For this review, take the finished solid that the model builds, in its own axes (mm). Face numbers are marked on the shaded views. A direction names the side the tool comes from. Coordinates: 2 decimals unless noted, no trailing zeros. Loops run counter-clockwise (first coordinate to the right, second up) from the corner with the lowest first, then second, coordinate; pieces in that order, holes last. Notation, with made-up numbers: (73.5, 33) -> (112.5, 33) arc R19 ccw to (112.5, 37) -> close; hole circle Ø9 at (79, -19.75). An arc over 180 degrees is marked (long way). Use a Markdown table: item, result.
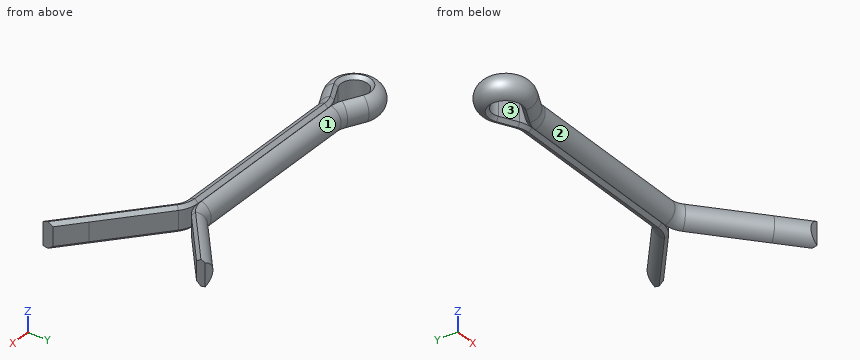
from build123d import *

# Parameters (mm, degrees)
ZKOSIT1_SIZE                  = 0.257142857
ZKOSIT2_SIZE                  = 0.45
ODEBRAT_VYSUNUT_M2_DEPTH      = 10
ODEBRAT_VYSUNUT_M2_DEPTH_BACK = 10
ODEBRAT_VYSUNUT_M3_DEPTH      = 15.066370457
ODEBRAT_VYSUNUT_M3_DEPTH_BACK = 15.066370457


with BuildPart() as part:
    # Táhnout po křivce1: sweep along a path in Skica1
    with BuildLine(Plane.XY) as t_hnout_po_k_ivce1_path:
        Line((10.498702419, 4.371053092), (6.640879802, 1.133955557))
        ThreePointArc((6.640879802, 1.133955557), (6.340112335, 0.960307379), (5.998092192, 0.9))
        Line((5.998092192, 0.9), (-5.998092192, 0.9))
        ThreePointArc((-5.998092192, 0.9), (-6.231322977, 0.927578589), (-6.451689409, 1.008793198))
        Line((-6.451689409, 1.008793198), (-7.621462583, 1.604172244))
        ThreePointArc((-7.621462583, 1.604172244), (-10.237937574, 0), (-7.621462583, -1.604172244))
        Line((-7.621462583, -1.604172244), (-6.451689409, -1.008793198))
        ThreePointArc((-6.451689409, -1.008793198), (-6.231322977, -0.927578589), (-5.998092192, -0.9))
        Line((-5.998092192, -0.9), (5.998092192, -0.9))
        ThreePointArc((5.998092192, -0.9), (6.340112335, -0.960307379), (6.640879802, -1.133955557))
        Line((6.640879802, -1.133955557), (10.498702419, -4.371053092))
        Line((10.498702419, -4.371053092), (12.413813527, -5.978022117))
    # Skica2 → Táhnout po křivce1 (sweep)
    with BuildSketch(Plane(origin=(10.498702419, 4.371053092, 0), x_dir=(0, 0, -1), z_dir=(0.7660444431189762, 0.6427876096865417, 0))):
        with BuildLine():
            Line((0.9, -0.9), (-0.9, -0.9))
            ThreePointArc((-0.9, -0.9), (0, 0), (0.9, -0.9))
        make_face()
    sweep(path=t_hnout_po_k_ivce1_path.line)

    # Zkosit1
    # the kernel refuses this chamfer: 0.257142857 mm, written as the material it takes off along each edge
    with BuildSketch(Plane(origin=(5.998092192, 0, 0.9), x_dir=(0, 0, -1), z_dir=(-1, 0, 0)), Plane(origin=(-5.998092192, 0, 0.9), x_dir=(0, 0, -1), z_dir=(1, 0, 0))) as zkosit1_piece_1:
        with BuildLine():
            Line((ZKOSIT1_SIZE, 0), (0.029314045, -0.227828812))
            ThreePointArc((0.029314045, -0.227828812), (0.007766605, -0.117981219), (0, 0))
            Line((0, 0), (ZKOSIT1_SIZE, 0))
        make_face()
    extrude(amount=11.996184384, mode=Mode.SUBTRACT)
    with BuildSketch(Plane(origin=(5.998092192, 0, -0.9), x_dir=(0, 0, 1), z_dir=(-1, 0, 0)), Plane(origin=(-5.998092192, 0, -0.9), x_dir=(0, 0, 1), z_dir=(1, 0, 0))) as zkosit1_piece_2:
        with BuildLine():
            Line((ZKOSIT1_SIZE, 0), (0.029314045, 0.227828812))
            ThreePointArc((0.029314045, 0.227828812), (0.007766605, 0.117981219), (0, 0))
            Line((0, 0), (ZKOSIT1_SIZE, 0))
        make_face()
    extrude(amount=11.996184384, mode=Mode.SUBTRACT)
    with BuildSketch(Plane(origin=(-5.998092192, 1.9, 0.9), x_dir=(0, -1, 0), z_dir=(1, 0, 0))) as zkosit1_piece_3:
        with BuildLine():
            Line((1.9, ZKOSIT1_SIZE), (1.672171188, 0.029314045))
            ThreePointArc((1.672171188, 0.029314045), (1.782018781, 0.007766605), (1.9, 0))
            Line((1.9, 0), (1.9, ZKOSIT1_SIZE))
        make_face()
    revolve(axis=Axis((-5.998092192, 1.9, 0.9), (0, 0, -1)), revolution_arc=26.974712985, mode=Mode.SUBTRACT)
    with BuildSketch(Plane(origin=(-5.998092192, 1.9, -0.9), x_dir=(0, -1, 0), z_dir=(1, 0, 0))) as zkosit1_piece_4:
        with BuildLine():
            Line((1.9, -ZKOSIT1_SIZE), (1.672171188, -0.029314045))
            ThreePointArc((1.672171188, -0.029314045), (1.782018781, -0.007766605), (1.9, 0))
            Line((1.9, 0), (1.9, -ZKOSIT1_SIZE))
        make_face()
    revolve(axis=Axis((-5.998092192, 1.9, -0.9), (0, 0, -1)), revolution_arc=26.974712985, mode=Mode.SUBTRACT)
    with BuildSketch(Plane(origin=(-6.859926905, 0.206707076, 0.9), x_dir=(0, 0, -1), z_dir=(-0.8912068023322748, 0.4535972172276652, 0)), Plane(origin=(-8.029700078, -0.802086122, 0.9), x_dir=(0, 0, -1), z_dir=(0.8912068023322748, 0.45359721722766544, 0))) as zkosit1_piece_5:
        with BuildLine():
            Line((ZKOSIT1_SIZE, 0), (0.029314045, -0.227828812))
            ThreePointArc((0.029314045, -0.227828812), (0.007766605, -0.117981219), (0, 0))
            Line((0, 0), (ZKOSIT1_SIZE, 0))
        make_face()
    extrude(amount=1.312572088, mode=Mode.SUBTRACT)
    with BuildSketch(Plane(origin=(-6.859926905, 0.206707076, -0.9), x_dir=(0, 0, 1), z_dir=(-0.8912068023322748, 0.4535972172276652, 0)), Plane(origin=(-8.029700078, -0.802086122, -0.9), x_dir=(0, 0, 1), z_dir=(0.8912068023322748, 0.45359721722766544, 0))) as zkosit1_piece_6:
        with BuildLine():
            Line((ZKOSIT1_SIZE, 0), (0.029314045, 0.227828812))
            ThreePointArc((0.029314045, 0.227828812), (0.007766605, 0.117981219), (0, 0))
            Line((0, 0), (ZKOSIT1_SIZE, 0))
        make_face()
    extrude(amount=1.312572088, mode=Mode.SUBTRACT)
    with BuildSketch(Plane(origin=(-8.437937574, 0, 0.9), x_dir=(0.4535972172277306, 0.8912068023322415, 0), z_dir=(0.8912068023322415, -0.4535972172277306, 0))) as zkosit1_piece_7:
        with BuildLine():
            Line((0.9, -ZKOSIT1_SIZE), (1.127828812, -0.029314045))
            ThreePointArc((1.127828812, -0.029314045), (1.017981219, -0.007766605), (0.9, 0))
            Line((0.9, 0), (0.9, -ZKOSIT1_SIZE))
        make_face()
    revolve(axis=Axis((-8.437937574, 0, 0.9), (0, 0, 1)), revolution_arc=233.94942597, mode=Mode.SUBTRACT)
    with BuildSketch(Plane(origin=(-8.437937574, 0, -0.9), x_dir=(0.4535972172277306, 0.8912068023322415, 0), z_dir=(0.8912068023322415, -0.4535972172277306, 0))) as zkosit1_piece_8:
        with BuildLine():
            Line((0.9, ZKOSIT1_SIZE), (1.127828812, 0.029314045))
            ThreePointArc((1.127828812, 0.029314045), (1.017981219, 0.007766605), (0.9, 0))
            Line((0.9, 0), (0.9, ZKOSIT1_SIZE))
        make_face()
    revolve(axis=Axis((-8.437937574, 0, -0.9), (0, 0, 1)), revolution_arc=233.94942597, mode=Mode.SUBTRACT)
    with BuildSketch(Plane(origin=(-5.998092192, -1.9, 0.9), x_dir=(-0.4535972172277067, 0.8912068023322537, 0), z_dir=(-0.8912068023322537, -0.4535972172277067, 0))) as zkosit1_piece_9:
        with BuildLine():
            Line((1.9, ZKOSIT1_SIZE), (1.672171188, 0.029314045))
            ThreePointArc((1.672171188, 0.029314045), (1.782018781, 0.007766605), (1.9, 0))
            Line((1.9, 0), (1.9, ZKOSIT1_SIZE))
        make_face()
    revolve(axis=Axis((-5.998092192, -1.9, 0.9), (0, 0, -1)), revolution_arc=26.974712985, mode=Mode.SUBTRACT)
    with BuildSketch(Plane(origin=(-5.998092192, -1.9, -0.9), x_dir=(-0.4535972172277067, 0.8912068023322537, 0), z_dir=(-0.8912068023322537, -0.4535972172277067, 0))) as zkosit1_piece_10:
        with BuildLine():
            Line((1.9, -ZKOSIT1_SIZE), (1.672171188, -0.029314045))
            ThreePointArc((1.672171188, -0.029314045), (1.782018781, -0.007766605), (1.9, 0))
            Line((1.9, 0), (1.9, -ZKOSIT1_SIZE))
        make_face()
    revolve(axis=Axis((-5.998092192, -1.9, -0.9), (0, 0, -1)), revolution_arc=26.974712985, mode=Mode.SUBTRACT)
    with BuildSketch(Plane(origin=(5.998092192, -1.9, 0.9), x_dir=(0, 1, 0), z_dir=(-1, 0, 0))) as zkosit1_piece_11:
        with BuildLine():
            Line((1.9, ZKOSIT1_SIZE), (1.672171188, 0.029314045))
            ThreePointArc((1.672171188, 0.029314045), (1.782018781, 0.007766605), (1.9, 0))
            Line((1.9, 0), (1.9, ZKOSIT1_SIZE))
        make_face()
    revolve(axis=Axis((5.998092192, -1.9, 0.9), (0, 0, -1)), revolution_arc=40, mode=Mode.SUBTRACT)
    with BuildSketch(Plane(origin=(5.998092192, -1.9, -0.9), x_dir=(0, 1, 0), z_dir=(-1, 0, 0))) as zkosit1_piece_12:
        with BuildLine():
            Line((1.9, -ZKOSIT1_SIZE), (1.672171188, -0.029314045))
            ThreePointArc((1.672171188, -0.029314045), (1.782018781, -0.007766605), (1.9, 0))
            Line((1.9, 0), (1.9, -ZKOSIT1_SIZE))
        make_face()
    revolve(axis=Axis((5.998092192, -1.9, -0.9), (0, 0, -1)), revolution_arc=40, mode=Mode.SUBTRACT)
    with BuildSketch(Plane(origin=(7.21938865, -0.444515558, 0.9), x_dir=(0, 0, -1), z_dir=(0.7660444431189773, -0.6427876096865403, 0)), Plane(origin=(13.498899837, -5.713651079, -0.9), x_dir=(0, 0, 1), z_dir=(-0.7660444431189773, 0.6427876096865401, 0))) as zkosit1_piece_13:
        with BuildLine():
            Line((ZKOSIT1_SIZE, 0), (0.029314045, -0.227828812))
            ThreePointArc((0.029314045, -0.227828812), (0.007766605, -0.117981219), (0, 0))
            Line((0, 0), (ZKOSIT1_SIZE, 0))
        make_face()
    extrude(amount=8.197319677, mode=Mode.SUBTRACT)
    with BuildSketch(Plane(origin=(11.58378873, 4.106682055, -0.9), x_dir=(0, 0, 1), z_dir=(-0.766044443118977, -0.6427876096865406, 0))) as zkosit1_piece_14:
        with BuildLine():
            Line((ZKOSIT1_SIZE, 0), (0.029314045, 0.227828812))
            ThreePointArc((0.029314045, 0.227828812), (0.007766605, 0.117981219), (0, 0))
            Line((0, 0), (ZKOSIT1_SIZE, 0))
        make_face()
    extrude(amount=5.697319677, mode=Mode.SUBTRACT)
    with BuildSketch(Plane(origin=(11.58378873, 4.106682055, 0.9), x_dir=(0, 0, -1), z_dir=(-0.766044443118977, -0.6427876096865406, 0))) as zkosit1_piece_15:
        with BuildLine():
            Line((ZKOSIT1_SIZE, 0), (0.029314045, -0.227828812))
            ThreePointArc((0.029314045, -0.227828812), (0.007766605, -0.117981219), (0, 0))
            Line((0, 0), (ZKOSIT1_SIZE, 0))
        make_face()
    extrude(amount=5.697319677, mode=Mode.SUBTRACT)
    with BuildSketch(Plane(origin=(5.998092192, 1.9, 0.9), x_dir=(0.6427876096865431, -0.7660444431189749, 0), z_dir=(0.7660444431189749, 0.6427876096865431, 0))) as zkosit1_piece_16:
        with BuildLine():
            Line((1.9, ZKOSIT1_SIZE), (1.672171188, 0.029314045))
            ThreePointArc((1.672171188, 0.029314045), (1.782018781, 0.007766605), (1.9, 0))
            Line((1.9, 0), (1.9, ZKOSIT1_SIZE))
        make_face()
    revolve(axis=Axis((5.998092192, 1.9, 0.9), (0, 0, -1)), revolution_arc=40, mode=Mode.SUBTRACT)
    with BuildSketch(Plane(origin=(5.998092192, 1.9, -0.9), x_dir=(0.6427876096865431, -0.7660444431189749, 0), z_dir=(0.7660444431189749, 0.6427876096865431, 0))) as zkosit1_piece_17:
        with BuildLine():
            Line((1.9, -ZKOSIT1_SIZE), (1.672171188, -0.029314045))
            ThreePointArc((1.672171188, -0.029314045), (1.782018781, -0.007766605), (1.9, 0))
            Line((1.9, 0), (1.9, -ZKOSIT1_SIZE))
        make_face()
    revolve(axis=Axis((5.998092192, 1.9, -0.9), (0, 0, -1)), revolution_arc=40, mode=Mode.SUBTRACT)

    # Zkosit2
    zkosit2_edges = [part.edges().sort_by_distance(p)[0] for p in [
        (12.992322376, -5.288582118, 0),
        (11.077211268, 3.681613094, 0),
    ]]
    chamfer(zkosit2_edges, length=ZKOSIT2_SIZE)

    # Skica5 → Odebrat vysunutím2 (cut, two sides: drawn at the far end of the back side and taken through both)
    with BuildSketch(Plane.XY.offset(-ODEBRAT_VYSUNUT_M2_DEPTH_BACK)):
        Polygon((10.787956844, 4.026333093), (10.15398242, 4.081798668), (10.498702419, 4.371053092), align=None)
    extrude(amount=ODEBRAT_VYSUNUT_M2_DEPTH + ODEBRAT_VYSUNUT_M2_DEPTH_BACK, mode=Mode.SUBTRACT)

    # Skica6 → Odebrat vysunutím3 (cut, two sides: drawn at the far end of the back side and taken through both)
    with BuildSketch(Plane.XY.offset(-ODEBRAT_VYSUNUT_M3_DEPTH_BACK)):
        Polygon((12.703067951, -5.633302117), (12.069093528, -5.688767692), (12.413813527, -5.978022117), align=None)
    extrude(amount=ODEBRAT_VYSUNUT_M3_DEPTH + ODEBRAT_VYSUNUT_M3_DEPTH_BACK, mode=Mode.SUBTRACT)


solid = part.part
(1) Take a section at A-A on x = 0.5. Write out the cut boundary in (y, z).
Found:
| item | result |
|---|---|
| outline | (-0.23, -0.87) -> (0, -0.64) -> (0.23, -0.87) arc R0.9 ccw to (0.23, 0.87) -> (0, 0.64) -> (-0.23, 0.87) arc R0.9 ccw to start |
(2) For the marked faces 1, 2 and 3, list the 3-axis set-ups (+Z, -Z, +X, -X, +Y, -Y) from which the entire face can be reached by the end or side of a thin tool; tool diameter is ignored.
Found:
| item | result |
|---|---|
| face 1 | +Y |
| face 2 | -Y |
| face 3 | +Z, -Z |
(3) For pin 1 Ø3 at (x, y) = (2, -2) entering from -Z; pin 2 Ø0.6 at (x, z) = (-0.5, 0) entering from +Y; pin 3 Ø4 at (x, y) = (9.5, -0.5) entering from -Z, all flat-tipped, find the tip position at first contact; note any pin that passes through.
Found:
| item | result |
|---|---|
| pin 1 | stops at z = -0.75 |
| pin 2 | stops at y = 0.9 |
| pin 3 | stops at z = -0.87 |
(4) For line 1 along X through (y, z) = (1, 0.3); line 2 along Y through (x, z) = (10.5, -0.6); line 3 along Y through (x, z) = (7.25, -0.55), list the stretches that pass through material, from the lowest coordinate up.
Found:
| item | result |
|---|---|
| line 1 | x = -9.87 to -6.55, 6.54 to 7.88 |
| line 2 | y = -4.07 to -3.2, 3.2 to 4.05 |
| line 3 | y = -1.4 to -0.47, 0.47 to 1.4 |
